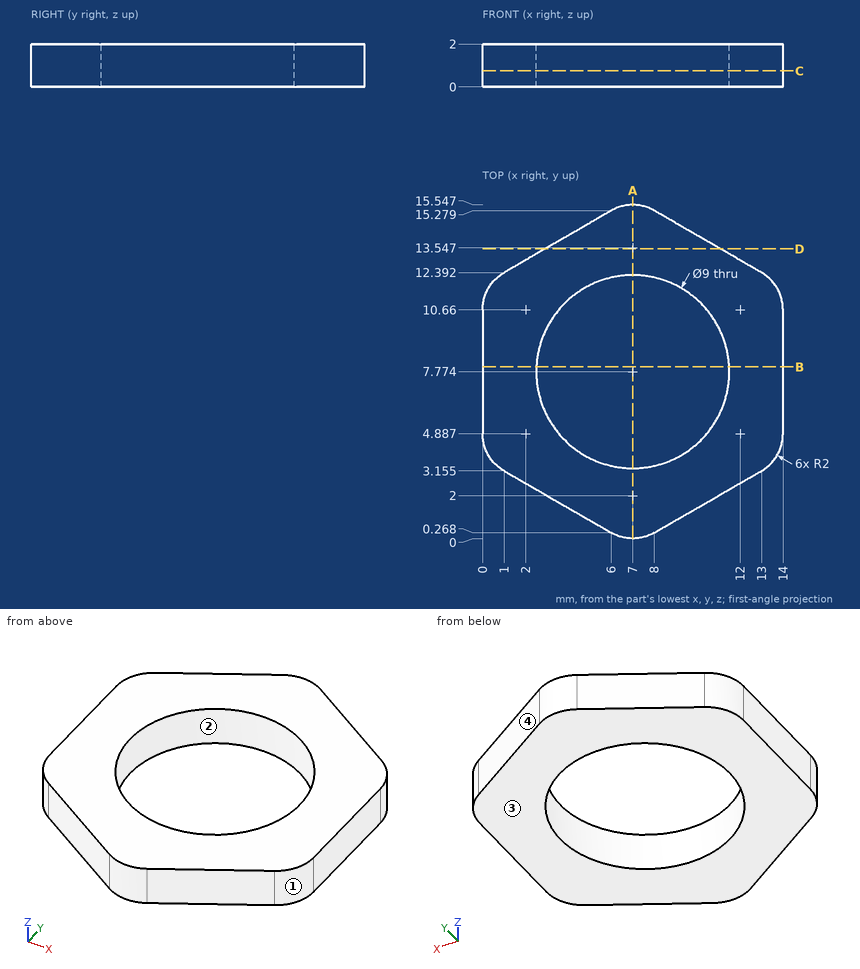
Here's the drawing with two shaded views (mm, measured from the low corner). I have some questions. Round coordinates to 2 decimals unless told otherwise and drop trailing zeros. Loops run counter-clockwise (first coordinate to the right, second up) from the corner with the lowest first, then second, coordinate; pieces in that order, holes last.
Item 1: Will these pins go through, and if not, where does the flat tip stop? pin 1 Ø1 at (x, z) = (7.5, 1.5) entering from +Y; pin 2 Ø1 at (x, z) = (10, 1) entering from -Y (1 decimal).
Item 2: Suppose I cut it at A-A, the plane x = 7. Write out the boundary of the cut face in (y, z).
Item 3: If we mould it in two halves opening along Y, with no side actions, what happens to the marked faces 1, 2, 3 and 4? For each: +Y half, -Y half, draft (parallel to the pull), parting line (faces both ways), or undercut.
Item 4: Suppose I cut it at D-D, the plane y = 13.5. Write out the boundary of the cut face in (x, z).
Item 5: Suppose I cut it at C-C, the plane z = 0.75. Write out the boundary of the cut face in (x, y) (1 decimal), then the cut area to 3 significant figures.
Item 6: Please list where these lines run through material, in increasing order: L1, parallel to Y at x = 7, z = 1.35; L2, parallel to X at y = 5, z = 1.7 (1 decimal); L3, parallel to Y at x = 5.5, z = 1.2 (1 decimal).
Item 7: Suppose I cut it at B-B, the plane y = 8. Write out the boundary of the cut face in (x, z) (1 decimal), then the cut area to 3 significant figures.
Reported:
1. pin 1: stops at y = 15.55
1. pin 2: stops at y = 1.1
2. outline: (0, 0) - (3.27, 0) - (3.27, 2) - (0, 2) - close; (12.27, 0) - (15.55, 0) - (15.55, 2) - (12.27, 2) - close
3. face 1: -Y half
3. face 2: undercut
3. face 3: draft
3. face 4: +Y half
4. outline: (2.92, 0) - (11.08, 0) - (11.08, 2) - (2.92, 2) - close
5. outline: (0, 4.9) arc R2 ccw to (1, 3.2) - (6, 0.3) arc R2 ccw to (8, 0.3) - (13, 3.2) arc R2 ccw to (14, 4.9) - (14, 10.7) arc R2 ccw to (13, 12.4) - (8, 15.3) arc R2 ccw to (6, 15.3) - (1, 12.4) arc R2 ccw to (0, 10.7) - close; hole circle Ø9 at (7, 7.8)
5. area: 105 mm2
6. L1: y = 0 to 3.27, 12.27 to 15.55
6. L2: x = 0 to 3.5, 10.5 to 14
6. L3: y = 0.6 to 3.5, 12 to 15
7. outline: (0, 0) - (2.5, 0) - (2.5, 2) - (0, 2) - close; (11.5, 0) - (14, 0) - (14, 2) - (11.5, 2) - close
7. area: 10.0 mm2
